Autodesk Inventor part; units mm, degrees
ref_plane "Work Plane1" through (0, 0, -406.4) normal (0, 0, 1) x (1, 0, 0)
ref_plane "YZ Plane" through (0, 0, 0) normal (1, 0, 0) x (0, 1, 0)
ref_plane "XZ Plane" through (0, 0, 0) normal (0, 1, 0) x (-1, 0, 0)
sketch "Sketch1" plane through (0, 0, 0) normal (0, 1, 0) x (-1, 0, 0)
  point P0 (0, 0)
sketch "Sketch2" plane through (0, 0, 0) normal (0, 1, 0) x (-1, 0, 0)
  line L0 (0, 0) -> (25.4, 0)
  line L1 (25.4, 0) -> (25.4, -812.8)
  line L2 (25.4, -812.8) -> (0, -812.8)
  line L3 (0, -812.8) -> (0, 0)
  dimension "d0" = 812.8
  dimension "d1" = 25.4
extrude "Extrusion1" add sketch "Sketch2" along normal blind 50.8
sketch "Sketch3" plane through (0, 0, 0) normal (1, 0, 0) x (0, 0, -1)
  circle A0 centre (133.35, 26.9875) radius 14.2875
  line L0 (0, 0) -> (0, 50.8)
  line L1 (0, 50.8) -> (812.8, 50.8)
  circle A1 centre (679.45, 26.9875) radius 14.2875
  line L2 (812.8, 0) -> (812.8, 50.8)
  line L3 (812.8, 0) -> (0, 0)
  circle A2 centre (406.4, 23.8125) radius 19.05
  point P0 (406.4, 50.8)
  point P1 (406.4, 0)
  point P2 (406.4, 0)
  dimension "d4" = 28.575
  dimension "d5" = 133.35
  dimension "d6" = 23.8125
  dimension "d7" = 28.575
  dimension "d8" = 133.35
  dimension "d9" = 26.9875
  dimension "d10" = 38.1
  dimension "d11" = 26.9875
extrude "Extrusion2" cut sketch "Sketch3" against normal through all contours A0 | A1 | A2
sketch "Sketch4" plane through (-25.4, 0, 0) normal (0, 0, 1) x (1, 0, 0)
  line L0 (0, 50.8) -> (25.4, 50.8)
  line L1 (25.4, 0) -> (25.4, 50.8)
  line L2 (25.4, 0) -> (0, 0)
  line L3 (0, 0) -> (0, 50.8)
  line L4 (22.225, 47.625) -> (3.175, 47.625)
  line L5 (3.175, 47.625) -> (3.175, 3.175)
  line L6 (3.175, 3.175) -> (22.225, 3.175)
  line L7 (22.225, 3.175) -> (22.225, 47.625)
  dimension "d15" = 3.175
extrude "Extrusion3" cut sketch "Sketch4" against normal up to surface (812.8 mm away) contours L7 L6 L5 L4
sketch "Sketch5" plane through (0, 0, 0) normal (1, 0, 0) x (0, 0, -1)
  circle A0 centre (679.45, 26.9875) radius 14.2875
  circle A1 centre (133.35, 26.9875) radius 14.2875
  circle A2 centre (406.4, 23.8125) radius 19.05
  line L0 (812.8, 0) -> (0, 0)
  line L1 (812.8, 0) -> (812.8, 50.8)
  line L2 (0, 50.8) -> (812.8, 50.8)
  line L3 (0, 0) -> (0, 50.8)
  line L4 (0, 50.8) -> (25.4, 50.8)
  line L5 (25.4, 50.8) -> (25.4, 0)
  line L6 (25.4, 0) -> (0, 0)
  line L7 (0, 0) -> (0, 50.8)
  line L8 (812.8, 0) -> (812.8, 50.8)
  line L9 (812.8, 0) -> (0, 0)
  line L10 (812.8, 50.8) -> (787.4, 50.8)
  line L11 (787.4, 50.8) -> (787.4, 0)
  line L12 (787.4, 0) -> (812.8, 0)
  line L13 (812.8, 0) -> (812.8, 50.8)
  dimension "d18" = 25.4
  dimension "d19" = 25.4
  dimension "d59" = 28.575
extrude "Extrusion4" cut sketch "Sketch5" against normal blind 25.4 contours L0 L11 L2 L1 | L0 L3 L2 L5
sketch "Sketch8" plane through (0, 0, -25.4) normal (1, 0, 0) x (0, 0, -1)
  point P0 (-25.4, 0)
sketch "Sketch9" plane through (0, 0, -25.4) normal (1, 0, 0) x (0, 0, -1)
  circle A0 centre (404.8252, 23.8125) radius 3.175
  circle A1 centre (381, 23.8125) radius 19.05
  line L0 (0, 50.8) -> (762, 50.8)
  circle A2 centre (357.1748, 23.8125) radius 3.175
  circle A3 centre (438.1754, 23.8125) radius 3.175
  circle A4 centre (323.8246, 23.8125) radius 3.175
  point P0 (-25.4, 0)
  point P1 (257.298, 23.8125)
  dimension "d61" = 6.35
  dimension "d62" = 23.8252
  dimension "d64" = 6.35
  dimension "d65" = 23.8252
  dimension "d67" = 6.35
  dimension "d69" = 6.35
  dimension "d71" = 57.1754
  dimension "d72" = 57.1754
extrude "Extrusion6" cut sketch "Sketch9" against normal blind 25.4 contours A0 | A2 | A3 | A4
sketch "Sketch11" plane through (-25.4, 0, -787.4) normal (-1, 0, 0) x (0, 0, 1)
  circle A0 centre (438.1754, 23.8125) radius 4.7625
  circle A1 centre (381, 23.8125) radius 19.05
  line L0 (0, 50.8) -> (762, 50.8)
  circle A2 centre (323.8246, 23.8125) radius 4.7625
  point P0 (787.4, 0)
  dimension "d85" = 9.525
  dimension "d86" = 57.1754
  dimension "d88" = 9.525
  dimension "d90" = 57.1754
extrude "Extrusion8" cut sketch "Sketch11" against normal blind 12.7 contours A0 | A2
sketch "Sketch12" plane through (-25.4, 0, -787.4) normal (-1, 0, 0) x (0, 0, 1)
  circle A0 centre (609.6, 19.05) radius 4.7625
  line L0 (762, 0) -> (0, 0)
  circle A1 centre (381, 23.8125) radius 19.05
  circle A2 centre (654.05, 26.9875) radius 14.2875
  point P0 (787.4, 0)
  dimension "d93" = 9.525
  dimension "d94" = 19.05
  dimension "d103" = 44.45
extrude "Extrusion9" cut sketch "Sketch12" against normal blind 12.7 contours A0
sketch "Sketch13" plane through (0, 0, -25.4) normal (1, 0, 0) x (0, 0, -1)
  circle A0 centre (152.4, 19.05) radius 1.905
  circle A1 centre (381, 23.8125) radius 19.05
  line L0 (762, 0) -> (0, 0)
  circle A2 centre (107.95, 26.9875) radius 14.2875
  point P0 (-25.4, 0)
  dimension "d98" = 3.81
  dimension "d100" = 19.05
  dimension "d104" = 44.45
extrude "Extrusion10" cut sketch "Sketch13" against normal blind 12.7 contours A0
ref_plane "Work Plane1" through (0, 0, -406.4) normal (0, 0, 1) x (1, 0, 0)
mirror "Mirror1" about plane through (0, 0, -406.4) normal (0, 0, 1) of "Extrusion10", "Extrusion9"
equation "\"d9\" = d11"
properties part number "2x1 20in Alluminum with Cal Drop.ver1-1111-2019"
Verification items for the finished model (mm, model axes). A direction names the side the tool comes from. Give positions to 0.01 mm unless a question says otherwise; leave off trailing zeros. Loops run counter-clockwise (first coordinate to the right, second up) from the corner with the lowest first, then second, coordinate; pieces in that order, holes last. Notation, with made-up numbers: (26.5, -13) - (83.5, -13) arc R19 ccw to (83.5, 1) - close; hole circle Ø8 at (-9.5, -11). An arc over 180 degrees is marked (long way). Write item = value, one per line. Start each with the question number.
Q1. Mould release check, pull along Z, two halves, no side actions. Record for faces 3 (the face through (-13, 47.625, -401)), 4 (the face through (-2, 26, -25.4)), 5 (the face through (-23.79, 27.616, -665.176)), 6 (the face through (-1.565, 39.035, -141.031)): released by +Z, released by -Z, zero draft, split by the parting line, or undercut.
Q2. Thickness scan on line 1 (X direction, y = 20, z = -196.5) (3 decimals); line 2 (Y direction, x = -16.75, z = -218) (3 decimals); line 3 (Z direction, x = -1.25, y = 28). Record the ranges inside material, lowest first.
Q3. Depth check by flat-ended pin: P1, Ø4, axis at y = 23.81, z = -430.23, coming from the +X side. Enter the tip coordinate at first touch or a pass-through.
Q4. Cross-section at A-A, the plane z = -679.45. Enter the section's corners in (x, y) (3 decimals), and give its area (3 significant figures).
Q5. Cross-section at B-B, the plane z = -338. Enter the section's corners in (x, y) (3 decimals), and give its area (3 significant figures).
Q6. Cross-section at C-C, the plane z = -139. Enter the section's corners in (x, y) (3 decimals).
Q7. Tool access check on faces 1 (the face through (-13, 3.175, -401)), 2 (the face through (0, 2, -412)). Record the directions out of +Z, -Z, +X, -X, +Y, -Y that give a thin tool (end or side, any length) a straight path to the whole face; none if there is none.
Answer key:
q1.face_3 = zero draft
q1.face_4 = released by +Z
q1.face_5 = undercut
q1.face_6 = undercut
q2.line_1 = -25.4 to -22.225, -3.175 to 0
q2.line_2 = 0 to 3.175, 47.625 to 50.8
q2.line_3 = -787.4 to -693.7, -665.2 to -424.98, -387.82 to -147.6, -119.1 to -25.4
q3.P1 = through
q4.outline = (-25.4, 0) - (0, 0) - (0, 12.7) - (-3.175, 12.7) - (-3.175, 3.175) - (-22.225, 3.175) - (-22.225, 12.7) - (-25.4, 12.7) - close; (-25.4, 41.275) - (-22.225, 41.275) - (-22.225, 47.625) - (-3.175, 47.625) - (-3.175, 41.275) - (0, 41.275) - (0, 50.8) - (-25.4, 50.8) - close
q4.area = 262 mm^2
q5.outline = (-25.4, 0) - (0, 0) - (0, 50.8) - (-25.4, 50.8) - close; hole (-22.225, 3.175) - (-3.175, 3.175) - (-3.175, 47.625) - (-22.225, 47.625) - close
q5.area = 444 mm^2
q6.outline = (-25.4, 0) - (0, 0) - (0, 13.865) - (-3.175, 13.865) - (-3.175, 3.175) - (-22.225, 3.175) - (-22.225, 13.865) - (-25.4, 13.865) - close; (-25.4, 40.11) - (-22.225, 40.11) - (-22.225, 47.625) - (-3.175, 47.625) - (-3.175, 40.11) - (0, 40.11) - (0, 50.8) - (-25.4, 50.8) - close
q7.face_1 = +Z, -Z
q7.face_2 = +Z, -Z, +X, +Y, -Y
